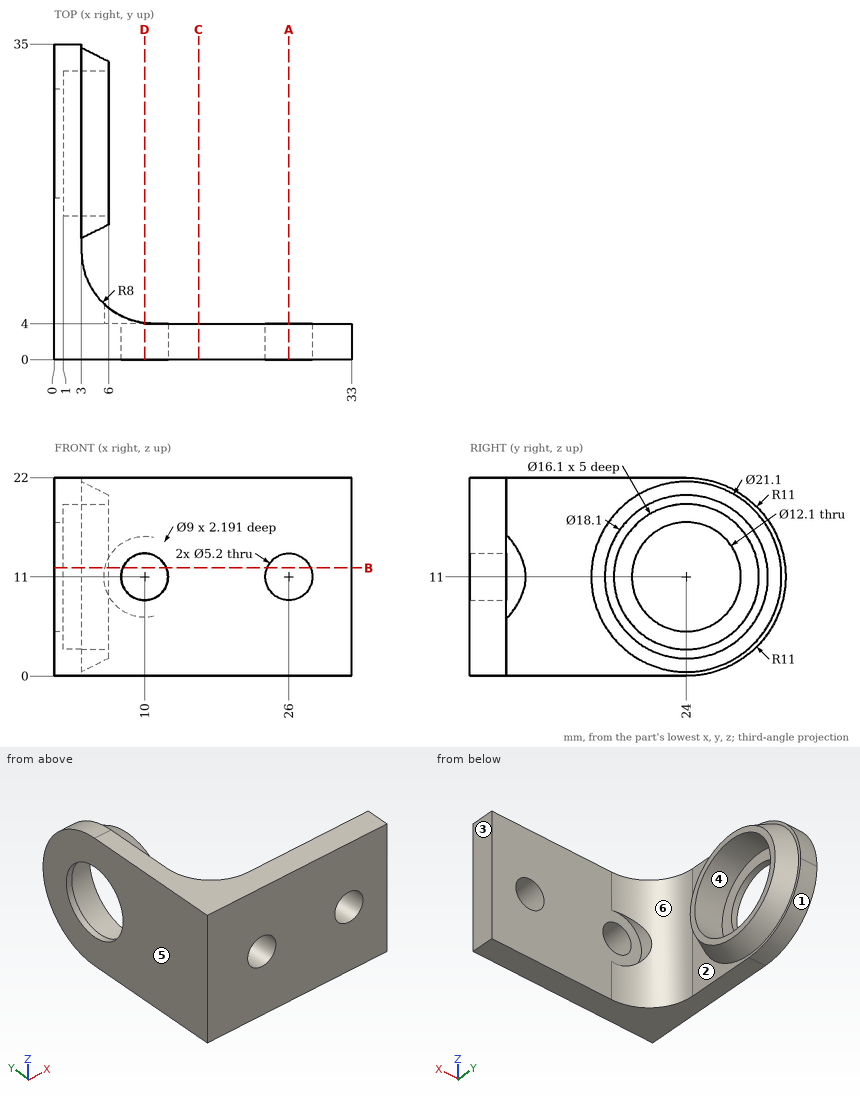
Here's the drawing with two shaded views (mm, measured from the low corner). I have some questions. A direction names the side the tool comes from. Coordinates: 2 decimals unless noted, no trailing zeros. Loops run counter-clockwise (first coordinate to the right, second up) from the corner with the lowest first, then second, coordinate; pieces in that order, holes last. Notation, with made-up numbers: M 56,38.5 L 66,38.5 A26 cw 66,73.5 Z; hole C 31.25,-40 d7. An arc over 180 degrees is marked long. Return JSON: item names as keys, results as strings. Group by question number.
Item 1: Imagine slicing it at B-B (z = 12). Give the number of separate pieces and of enclosed holes in the cut face, and give its area (3 significant figures).
Item 2: Imagine slicing it at C-C (x = 16). Please give me the cut outline in (y, z), and give its area (3 significant figures).
Item 3: Imagine slicing it at D-D (x = 10). Please give me the cut outline in (y, z).
Item 4: I'm going to push flat-ended pins straight in: pin 1 Ø1 at (y, z) = (15.5, 14) entering from +X; pin 2 Ø3 at (x, z) = (26, 11) entering from -Y; pin 3 Ø6 at (x, z) = (3.5, 10) entering from +Y; pin 4 Ø6 at (y, z) = (9, 11.5) entering from +X. Where does each tip first touch, or does it pass through?
Item 5: On a 3-axis mill with a long thin cutter (end or side, diameter ignored), from which of +Z, -Z, +X, -X, +Y, -Y can I reach the whole of each face in a straight line? I mean the marked faces 4, 5 and 6. Say none if no direction works.
Item 6: If I drill on L1, parallel to Z at x = 26, y = 1.65; L2, parallel to Y at x = 18, z = 19.5; L3, parallel to X at y = 12, z = 16.75, over which ranges is the centre line in solid material (lowest first)? Write a range as from..to.
Item 7: Thinking about a two-plate mould opening in Y: for the marked faces 1, 2 and 3, which applies, released by +Y, released by -Y, zero draft, split by the parting line, or undercut?
Item 8: Imagine slicing it at A-A (x = 26). Please give me the cut outline in (y, z), and give its area (3 significant figures).
Verdict:
{
 "1": {"separate pieces": "4", "enclosed holes": "0", "area": "163 mm^2"},
 "2": {"outline": "M 0,0 L 4,0 L 4,22 L 0,22 Z", "area": "88.0 mm^2"},
 "3": {"outline": "M 0,0 L 4.06,0 L 4.06,6.5 L 4,6.5 L 4,8.4 L 0,8.4 Z; M 0,13.6 L 4,13.6 L 4,15.5 L 4.06,15.5 L 4.06,22 L 0,22 Z"},
 "4": {"pin 1": "stops at x = 6", "pin 2": "passes through", "pin 3": "stops at y = 35", "pin 4": "stops at x = 5.64"},
 "5": {"face 4": "+X", "face 5": "+Z, -Z, -X, +Y, -Y", "face 6": "+Z, -Z, +X"},
 "6": {"L1": "z = 0..8.4, 13.6..22", "L2": "y = 0..4", "L3": "x = 0..3"},
 "7": {"face 1": "released by +Y", "face 2": "undercut", "face 3": "zero draft"},
 "8": {"outline": "M 0,0 L 4,0 L 4,8.4 L 0,8.4 Z; M 0,13.6 L 4,13.6 L 4,22 L 0,22 Z", "area": "67.2 mm^2"}
}
